Source: CAD feature listing. Evaluate the final solid. Frame: model axes, mm. Face numbers are marked on the shaded views. A direction names the side the tool comes from. Round coordinates to 2 decimals unless told otherwise and drop trailing zeros. Write each loop counter-clockwise with the first axis right and the second up, starting at its lowest first coordinate (ties: lowest second). Pieces come first, ordered by that corner, then holes. Notation, with made-up numbers: M -10,16 L 43,16 A31 ccw 43,55 Z; hole C -14.75,-38 d2. An arc over 180 degrees is marked long. Use a Markdown table: item, result.
```python
from build123d import *

# Parameters (mm, degrees)
SKETCH_1_W           = 23
SKETCH_1_H           = 12.2
EXTRUDE_1_DEPTH      = 24
EXTRUDE_2_DEPTH      = 4.6
EXTRUDE_2_DEPTH_BACK = 28.6
SKETCH_2_W           = 2
SKETCH_2_H           = 12.2
SKETCH_3_R           = 5.5
EXTRUDE_3_DEPTH      = 4.6


with BuildPart() as part:
    # 草图1 → 凸台-拉伸1 (new body)
    with BuildSketch(Plane.XY):
        with Locations((11.5, 6.1)):
            Rectangle(SKETCH_1_W, SKETCH_1_H)
    extrude(amount=EXTRUDE_1_DEPTH)

    # 草图2 → 凸台-拉伸2 (add, two sides: drawn at the far end of the back side and taken through both)
    with BuildSketch(Plane.XY.offset(24).offset(-EXTRUDE_2_DEPTH_BACK)):
        with Locations((5, 6.1)):
            Rectangle(SKETCH_2_W, SKETCH_2_H)
    extrude(amount=EXTRUDE_2_DEPTH + EXTRUDE_2_DEPTH_BACK)

    # 草图3 → 凸台-拉伸3 (add)
    with BuildSketch(Plane.ZY):
        with Locations((6, 6.1)):
            Circle(SKETCH_3_R)
    extrude(amount=EXTRUDE_3_DEPTH)


solid = part.part
```
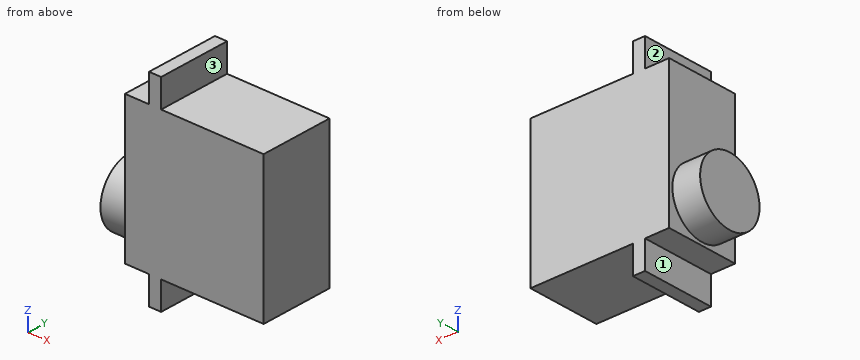
Q1. Line query: L1, parallel to Z at x = 9.25, y = 6; L2, parallel to X at y = 6.5, z = 24.5; L3, parallel to X at y = 1, z = 21.5. Output: solid intervals per line, ascending.
Results are:
| item | result |
|---|---|
| L1 | 0 to 24 |
| L2 | 4 to 6 |
| L3 | 0 to 23 |
Q2. Section A-A on z = 6. Return loops of the section in (x, y).
Results are:
| item | result |
|---|---|
| outline | M -4.6,0.6 L 0,0.6 L 0,0 L 23,0 L 23,12.2 L 0,12.2 L 0,11.6 L -4.6,11.6 Z |
Q3. Reachability of the marked faces 1, 2 and 3 from +Z, -Z, +X, -X, +Y, -Y: full face, straight path, thin tool, end or side. Return the list, or none.
Results are:
| item | result |
|---|---|
| face 1 | -Z, -X, +Y, -Y |
| face 2 | +Z, -X, +Y, -Y |
| face 3 | +Z, +X, +Y, -Y |
Q4. First-contact query: pin 1 Ø1.4 at (y, z) = (7.5, 25.5) entering from +X; pin 2 Ø4 at (y, z) = (7, 22.5) entering from -X; pin 3 Ø3 at (x, y) = (-1, 5.5) entering from +Z. Flat tips, straight axial feed; report the tip coordinate or a pass-through.
Results are:
| item | result |
|---|---|
| pin 1 | x = 6 |
| pin 2 | x = 0 |
| pin 3 | z = 24 |
Q5. Section C-C on x = 2.5. Return loops of the section in (y, z), plus the area to 3 significant figures.
Results are:
| item | result |
|---|---|
| outline | M 0,0 L 12.2,0 L 12.2,24 L 0,24 Z |
| area | 293 mm^2 |
Q6. Section B-B on y = 6.1. Return loops of the section in (x, z).
Results are:
| item | result |
|---|---|
| outline | M -4.6,0.5 L 0,0.5 L 0,0 L 4,0 L 4,-4.6 L 6,-4.6 L 6,0 L 23,0 L 23,24 L 6,24 L 6,28.6 L 4,28.6 L 4,24 L 0,24 L 0,11.5 L -4.6,11.5 Z |
Q7. Section D-D on y = 3. Return loops of the section in (x, z).
Results are:
| item | result |
|---|---|
| outline | M -4.6,1.46 L 0,1.46 L 0,0 L 4,0 L 4,-4.6 L 6,-4.6 L 6,0 L 23,0 L 23,24 L 6,24 L 6,28.6 L 4,28.6 L 4,24 L 0,24 L 0,10.54 L -4.6,10.54 Z |
